from build123d import *

# Parameters (mm, degrees)
F0_R     = 1.6002
F0_R_2   = 3.3782
F0_W     = 44.8
F0_H     = 22
F0_R_3   = 8.873689
F0_R_4   = 1.0033
F1_DEPTH = 6


with BuildPart() as f1:
    # F0 (on Top) → F1 (new body)
    with BuildSketch(Plane.XY):
        Polygon((155.197096, 268.007227), (-111.502904, 268.007227), (-111.502904, -176.492773), (-73.402904, -176.492773), (-73.402904, -138.392773), (-67.402904, -138.392773), (-67.402904, -176.492773), (111.097096, -176.492773), (111.097096, -138.392773), (117.097096, -138.392773), (117.097096, -176.492773), (155.197096, -176.492773), align=None)
        with Locations((-22.602904, -31.712773)):
            Circle(F0_R, mode=Mode.SUBTRACT)
        with Locations((28.197096, -87.592773)):
            Circle(F0_R, mode=Mode.SUBTRACT)
        with Locations((117.097096, -31.712773)):
            Circle(F0_R_2, mode=Mode.SUBTRACT)
        with Locations((15.497096, 256.577227)):
            Circle(F0_R, mode=Mode.SUBTRACT)
        with Locations((120.097096, 146.581596)):
            Rectangle(F0_W, F0_H, mode=Mode.SUBTRACT)
        with Locations((129.797096, 104.177227)):
            Circle(F0_R, mode=Mode.SUBTRACT)
        with Locations((40.547096, 158.366844)):
            Circle(F0_R_3, mode=Mode.SUBTRACT)
        with Locations((28.297096, 212.476226)):
            Circle(F0_R_4, mode=Mode.SUBTRACT)
        with BuildLine():
            ThreePointArc((32.647096, 227.176226), (32.939989, 227.883333), (33.647096, 228.176226))
            Line((33.647096, 228.176226), (58.947096, 228.176226))
            ThreePointArc((58.947096, 228.176226), (59.654203, 227.883333), (59.947096, 227.176226))
            Line((59.947096, 227.176226), (59.947096, 197.776226))
            ThreePointArc((59.947096, 197.776226), (59.654203, 197.069119), (58.947096, 196.776226))
            Line((58.947096, 196.776226), (33.647096, 196.776226))
            ThreePointArc((33.647096, 196.776226), (32.939989, 197.069119), (32.647096, 197.776226))
            Line((32.647096, 197.776226), (32.647096, 227.176226))
        make_face(mode=Mode.SUBTRACT)
        with Locations((64.297096, 212.476226)):
            Circle(F0_R_4, mode=Mode.SUBTRACT)
        with Locations((120.272096, 177.736496)):
            Circle(F0_R, mode=Mode.SUBTRACT)
        with Locations((120.272096, 225.234496)):
            Circle(F0_R, mode=Mode.SUBTRACT)
        with Locations((129.797096, 256.577227)):
            Circle(F0_R, mode=Mode.SUBTRACT)
    extrude(amount=F1_DEPTH)


solid = f1.part
Here's how the part is built. I have some questions about the finished solid (model axes, mm). Give positions to 0.01 mm unless a question says otherwise; leave off trailing zeros. Use a Markdown table: item, result. Add a question column.
Item 1: Imagine slicing it at A-A on z = 1.55. Give the number of separate pieces and of enclosed holes in the cut face, plus the area to 3 significant figures.
Item 2: Will these pins go through, and if not, where does the flat tip stop? pin 1 (3 mm diameter, centred on x = 28.2, y = -87.59, fed in from +Z); pin 2 (2 mm diameter, centred on x = 35, y = -6, fed in from -Z); pin 3 (3 mm diameter, centred on x = 113, z = 4.5, fed in from -Y).
Item 3: If we mould it in two halves opening along X, with no side actions, what happens to faces 1 (the face through (20, 49, 6)), 2 (the face through (38.623, 149.704, 2.958))? For each: pulls with the +X half, pulls with the -X half, needs draft (parallel to the pull), parting line crosses it, or undercut.
Item 4: I need wall thicknesses on line 1 (X direction, y = -150.5, z = 0.8); line 2 (Y direction, x = 133, z = 5.7); line 3 (X direction, y = 211, z = 2.65). Which ranges of each line are inside material? Lowest first, please.
Data:
| question | item | result |
|---|---|---|
| 1 | separate pieces | 1 |
| 1 | enclosed holes | 13 |
| 1 | area | 116,000 mm² |
| 2 | pin 1 | passes through |
| 2 | pin 2 | stops at z = 0 |
| 2 | pin 3 | stops at y = -138.39 |
| 3 | face 1 | needs draft |
| 3 | face 2 | undercut |
| 4 | line 1 | x = -111.5 to -73.4, -67.4 to 111.1, 117.1 to 155.2 |
| 4 | line 2 | y = -176.49 to 135.58, 157.58 to 268.01 |
| 4 | line 3 | x = -111.5 to 32.65, 59.95 to 155.2 |
